The drawing under review shows one solid part. Ordinate dimensions are in mm from its lowest x, y, z. Coordinates: 2 decimals unless noted, no trailing zeros. Write each loop counter-clockwise with the first axis right and the second up, starting at its lowest first coordinate (ties: lowest second). Pieces come first, ordered by that corner, then holes. Notation, with made-up numbers: (-23, -23) - (14, -23) arc R28 cw to (14, 3) - close; hole circle Ø5 at (40, 64). An arc over 180 degrees is marked (long way). Put each result on its own line as item: value. Start each with the question number.
Item 1: Consider section A-A on z = 3.45. Give the boundary of the cut face in (x, y) (1 decimal).
Item 2: For pin 1 (2 mm diameter, centred on x = 39, z = 3.5, fed in from -Y); pin 2 (0.6 mm diameter, centred on y = 26, z = 3, fed in from +X); pin 3 (2 mm diameter, centred on y = 35.5, z = 4, fed in from -X), all flat-tipped, find the tip position at first contact; note any pin that passes through.
Item 3: To check wall thickness, follow L1, parallel to Y at x = 38, z = 2.65 (1 decimal); L2, parallel to X at y = 53, z = 2.95; L3, parallel to X at y = 68, z = 3.9 (1 decimal). State the ranges of each line that lie inside material, in increasing order. Write a range as [from, to].
Item 4: Consider section B-B on y = 45. Give the boundary of the cut face in (x, z).
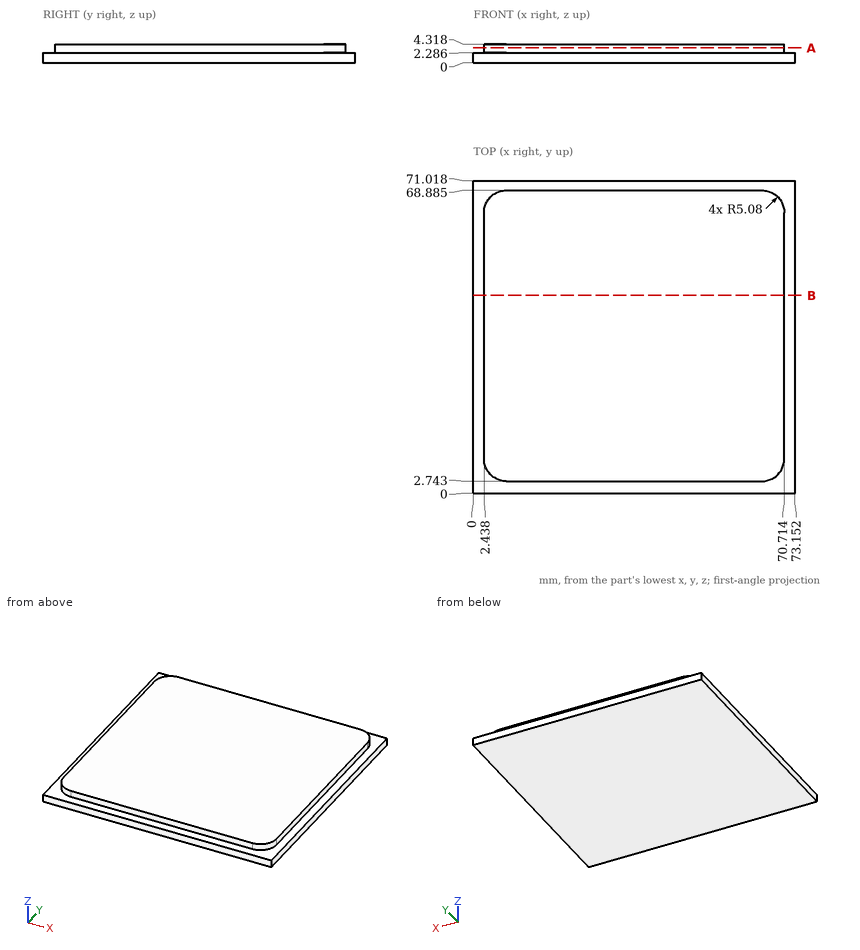
Report:
1. outline: (2.4, 7.8) arc R5.1 ccw to (7.5, 2.7) - (65.6, 2.7) arc R5.1 ccw to (70.7, 7.8) - (70.7, 63.8) arc R5.1 ccw to (65.6, 68.9) - (7.5, 68.9) arc R5.1 ccw to (2.4, 63.8) - close
2. pin 1: y = 2.74
2. pin 2: x = 70.71
2. pin 3: x = 2.44
3. L1: [2.7, 68.9]
3. L2: [2.44, 70.71]
3. L3: [4.7, 68.5]
4. outline: (0, 0) - (73.15, 0) - (73.15, 2.29) - (70.71, 2.29) - (70.71, 4.32) - (2.44, 4.32) - (2.44, 2.29) - (0, 2.29) - close
